Autodesk Inventor part; units mm, degrees
ref_plane "YZ Plane" through (0, 0, 0) normal (1, 0, 0) x (0, 1, 0)
ref_plane "XZ Plane" through (0, 0, 0) normal (0, 1, 0) x (-1, 0, 0)
ref_plane "XY Plane" through (0, 0, 0) normal (0, 0, 1) x (1, 0, 0)
sketch "Sketch1" plane through (0, 0, 0) normal (0, 1, 0) x (-1, 0, 0)
  circle A0 centre (12.7, 0) radius 38.1
  circle A1 centre (0, 0) radius 88.9
  circle A2 centre (0, 98.425) radius 9.525
  arc A3 (9.1574, 101.0457) -> (24.7665, 85.3805) centre (31.1351, 107.3355) ccw
  arc A4 (-24.7665, 85.3805) -> (-9.1574, 101.0457) centre (-31.1351, 107.3355) ccw
  circle A5 centre (-98.425, 0) radius 9.525
  circle A6 centre (0, -98.425) radius 9.525
  circle A7 centre (98.425, 0) radius 9.525
  arc A8 (85.3805, 24.7665) -> (101.0457, 9.1574) centre (107.3355, 31.1351) ccw
  arc A9 (24.7665, -85.3805) -> (9.1574, -101.0457) centre (31.1351, -107.3355) ccw
  arc A10 (-9.1574, -101.0457) -> (-24.7665, -85.3805) centre (-31.1351, -107.3355) ccw
  arc A11 (-85.3805, -24.7665) -> (-101.0457, -9.1574) centre (-107.3355, -31.1351) ccw
  arc A12 (-101.0457, 9.1574) -> (-85.3805, 24.7665) centre (-107.3355, 31.1351) ccw
  arc A13 (101.0457, -9.1574) -> (85.3805, -24.7665) centre (107.3355, -31.1351) ccw
  line L0 (98.425, 0) -> (88.9, 0)
  line L1 (0, 98.425) -> (0, 88.9)
  line L2 (0, -98.425) -> (0, -88.9)
  line L3 (-98.425, 0) -> (-88.9, 0)
  line L4 (12.7, 0) -> (0, 0)
  dimension "d20" = 177.8
  dimension "d0" = 76.2
  dimension "d2" = 19.05
  dimension "d3" = 22.86
  dimension "d21" = 12.7
extrude "Extrusion1" add sketch "Sketch1" along normal blind 6.35
sketch "Sketch3" plane through (0, 6.35, 0) normal (0, 1, 0) x (1, 0, 0)
  circle A0 centre (-12.7, 0) radius 38.1
  arc A1 (101.0457, -9.1574) -> (101.0457, 9.1574) centre (98.425, 0) ccw
  arc A2 (101.0457, -9.1574) -> (85.3805, -24.7665) centre (107.3355, -31.1351) ccw
  arc A3 (24.7665, -85.3805) -> (85.3805, -24.7665) centre (0, 0) ccw
  arc A4 (24.7665, -85.3805) -> (9.1574, -101.0457) centre (31.1351, -107.3355) ccw
  arc A5 (-9.1574, -101.0457) -> (9.1574, -101.0457) centre (0, -98.425) ccw
  arc A6 (-9.1574, -101.0457) -> (-24.7665, -85.3805) centre (-31.1351, -107.3355) ccw
  arc A7 (-85.3805, -24.7665) -> (-24.7665, -85.3805) centre (0, 0) ccw
  arc A8 (-85.3805, -24.7665) -> (-101.0457, -9.1574) centre (-107.3355, -31.1351) ccw
  arc A9 (-101.0457, 9.1574) -> (-101.0457, -9.1574) centre (-98.425, 0) ccw
  arc A10 (-101.0457, 9.1574) -> (-85.3805, 24.7665) centre (-107.3355, 31.1351) ccw
  arc A11 (-24.7665, 85.3805) -> (-85.3805, 24.7665) centre (0, 0) ccw
  arc A12 (-24.7665, 85.3805) -> (-9.1574, 101.0457) centre (-31.1351, 107.3355) ccw
  arc A13 (9.1574, 101.0457) -> (-9.1574, 101.0457) centre (0, 98.425) ccw
  arc A14 (9.1574, 101.0457) -> (24.7665, 85.3805) centre (31.1351, 107.3355) ccw
  arc A15 (85.3805, 24.7665) -> (24.7665, 85.3805) centre (0, 0) ccw
  arc A16 (85.3805, 24.7665) -> (101.0457, 9.1574) centre (107.3355, 31.1351) ccw
hole "Hole1" at (98.425, 6.35, 0) at (0, 6.35, 98.425) at (-98.425, 6.35, 0) at (0, 6.35, -98.425) direction (0, -1, 0) diameter 6.5278 depth 12.2936 tip angle 118
sketch "Sketch6" plane through (0, 0, 0) normal (0, -1, 0) x (1, 0, 0)
  circle A0 centre (-12.7, 0) radius 38.1
  circle A1 centre (-12.7, 0) radius 50
  circle A2 centre (-12.7, 0) radius 69.85
  circle A3 centre (-12.7, 0) radius 60.325
  line L0 (-12.7, 0) -> (-12.7, 60.325)
  circle A4 centre (-12.7, 0) radius 60.325
  circle A5 centre (-12.7, 0) radius 60.325
  circle A6 centre (-12.7, 0) radius 60.325
  circle A7 centre (-12.7, 0) radius 60.325
  circle A8 centre (-12.7, 0) radius 60.325
  point P0 (0, 0)
  point P1 (39.543, 30.1625)
  point P2 (39.543, -30.1625)
  point P3 (-12.7, -60.325)
  point P4 (-64.943, -30.1625)
  point P5 (-64.943, 30.1625)
  dimension "d22" = 100
  dimension "d27" = 360
  dimension "d36" = 139.7
  dimension "d37" = 9.525
hole "Hole2" at (-12.7, 0, 60.325) at (39.543, 0, 30.1625) at (39.543, 0, -30.1625) at (-12.7, 0, -60.325) at (-64.943, 0, -30.1625) at (-64.943, 0, 30.1625) direction (0, 1, 0) diameter 6.5278 depth 12.2936 tip angle 118
sketch "Sketch8" plane through (0, 6.35, 0) normal (0, 1, 0) x (1, 0, 0)
  circle A0 centre (-12.7, 0) radius 38.1
  circle A1 centre (-12.7, 0) radius 76.2
  circle A2 centre (-12.7, 0) radius 88.9
  arc A3 (38.2909, 72.8226) -> (31.0065, 62.4194) centre (34.6487, 67.621) ccw
  arc A4 (31.0065, -62.4194) -> (38.2909, -72.8226) centre (34.6487, -67.621) ccw
  line L0 (2.6706, 21.8863) -> (60.2892, 21.8863)
  line L1 (-12.7, 0) -> (34.6487, 67.621)
  line L2 (34.6487, -67.621) -> (-12.7, 0)
  arc A5 (73.1708, -23.009) -> (60.9035, -19.722) centre (67.0372, -21.3655) ccw
  arc A6 (60.9035, 19.722) -> (73.1708, 23.009) centre (67.0372, 21.3655) ccw
  line L3 (-12.7, 0) -> (67.0372, 21.3655)
  line L4 (-12.7, 0) -> (67.0372, -21.3655)
  circle A7 centre (-12.7, 0) radius 38.1
  point P0 (0, 0)
  dimension "d38" = 38.1
  dimension "d39" = 12.7
  dimension "d40" = 55
  dimension "d41" = 55
  dimension "d42" = 40
  dimension "d43" = 40
extrude "Extrusion3" cut sketch "Sketch8" against normal blind 25.4 contours A1 A3 A2 A6 | A5 A2 A4 A1
properties part number "LargeBearingPlate" material "Stainless Steel"
Verification items for the finished model (mm, model axes). A direction names the side the tool comes from. Give positions to 0.01 mm unless a question says otherwise; leave off trailing zeros. Write each loop counter-clockwise with the first axis right and the second up, starting at its lowest first coordinate (ties: lowest second). Pieces come first, ordered by that corner, then holes. Notation, with made-up numbers: (-10.75, 72.25) -> (-0.75, 72.25) arc R11 cw to (-0.75, 77.25) -> close; hole circle Ø8 at (30.5, 74.25). An arc over 180 degrees is marked (long way). Use CSV: the item, a comma, the result in double quotes.
(1) Go/stop test with flat-tipped pins: pin 1 (1.5 mm diameter, centred on y = 2, z = -77, fed in from +X); pin 2 (2 mm diameter, centred on x = 81.5, y = 5.5, fed in from +Z); pin 3 (6 mm diameter, centred on x = -12.7, z = -60.325, fed in from +Y); pin 4 (1 mm diameter, centred on y = 2.5, z = -54, fed in from -X). Record where each tip stops, or that it passes through.
Derived:
pin 1,"stops at x = 45.71"
pin 2,"stops at z = 37.72"
pin 3,"passes through"
pin 4,"stops at x = -71"
(2) Set-up check for faces 1 (the cylindrical face through (-107.95, 3.13, 0.17)), 2 (the cylindrical face through (59.87, 3.22, 51.35)): record each of +Z, -Z, +X, -X, +Y, -Y from which the full face is reachable in a straight line by a thin tool's end or side.
Derived:
face 1,"-X, +Y, -Y"
face 2,"+Y, -Y"
(3) Sectioned sample at C-C (x = 46). Record the cut outline in (y, z), plus the area to 3 significant figures.
Derived:
outline,"(0, -76.07) -> (6.35, -76.07) -> (6.35, -66.76) -> (0, -66.76) -> close; (0, -48.59) -> (6.35, -48.59) -> (6.35, 48.59) -> (0, 48.59) -> close; (0, 66.76) -> (6.35, 66.76) -> (6.35, 76.07) -> (0, 76.07) -> close"
area,"735 mm^2"
(4) Sectioned sample at A-A (z = 0). Record the cut outline in (x, y), plus the area to 3 significant figures.
Derived:
outline,"(-107.95, 0) -> (-101.69, 0) -> (-101.69, 6.35) -> (-107.95, 6.35) -> close; (-95.16, 0) -> (-50.8, 0) -> (-50.8, 6.35) -> (-95.16, 6.35) -> close; (25.4, 0) -> (95.16, 0) -> (95.16, 6.35) -> (25.4, 6.35) -> close; (101.69, 0) -> (107.95, 0) -> (107.95, 6.35) -> (101.69, 6.35) -> close"
area,"804 mm^2"
(5) Sectioned sample at B-B (x = -12.7). Record the cut outline in (y, z), plus the area to 3 significant figures.
Derived:
outline,"(0, -93.82) -> (6.35, -93.82) -> (6.35, -63.59) -> (0, -63.59) -> close; (0, -57.06) -> (6.35, -57.06) -> (6.35, -38.1) -> (0, -38.1) -> close; (0, 38.1) -> (6.35, 38.1) -> (6.35, 57.06) -> (0, 57.06) -> close; (0, 63.59) -> (6.35, 63.59) -> (6.35, 93.82) -> (0, 93.82) -> close"
area,"625 mm^2"
(6) Sectioned sample at D-D (x = -40.5). Record the cut outline in (y, z).
Derived:
outline,"(0, -79.14) -> (6.35, -79.14) -> (6.35, -26.05) -> (0, -26.05) -> close; (0, 26.05) -> (6.35, 26.05) -> (6.35, 79.14) -> (0, 79.14) -> close"
(7) Material ranges on L1, parallel to Z at x = 34.5, y = 0.5; L2, parallel to Z at x = 68, y = 4.75; L3, parallel to X at y = 3.75, z = -2, recorded low to high.
Derived:
L1,"z = -81.93 to -73.97, -59.82 to 59.82, 73.97 to 81.93"
L2,"z = -57.26 to -37.29, -15.09 to 15.09, 37.29 to 57.26"
L3,"x = -107.74 to -101, -95.85 to -50.75, 25.35 to 95.85, 101 to 107.74"
(8) Release check for a two-part mould opening along Z. For faces 3 (the cylindrical face through (-13.68, 3.22, -63.44)), 4 (the cylindrical face through (-0.17, 3.13, -107.95)), 5 (the cylindrical face through (14.828, 3.131, 91.315)) record: +Z half, -Z half, draft (parallel to the pull), parting line (faces both ways), or undercut.
Derived:
face 3,"undercut"
face 4,"-Z half"
face 5,"+Z half"
